Autodesk Inventor part; units mm, degrees
ref_plane "Work Plane1" through (42.6466, 0, 0) normal (1, 0, 0) x (0, 1, 0)
ref_plane "Work Plane2" through (-42.6466, 0, 0) normal (1, 0, 0) x (0, 1, 0)
ref_plane "Work Plane3" through (0, 0, -42.6466) normal (0, 0, 1) x (1, 0, 0)
sketch "Sketch1" plane through (0, 0, 0) normal (0, 0, 1) x (1, 0, 0)
  line L0 (17.5514, 0) -> (46.0756, 0)
  line L1 (46.0756, 0) -> (46.0756, 12.7)
  line L2 (46.0756, 12.7) -> (0, 12.7)
  line L3 (0, 12.7) -> (0, 0)
  line L4 (17.5514, 12.7) -> (17.5514, 0)
  line L5 (46.0756, 8.9662) -> (42.3672, 8.9662)
  line L6 (42.3672, 7.747) -> (42.3672, 0)
  line L7 (46.0756, 7.747) -> (42.3672, 7.747)
  line L8 (46.0756, 8.9662) -> (42.3672, 7.747)
  line L9 (0, 11.1252) -> (0, 12.7)
  line L10 (17.5514, 0) -> (23.85, 0)
  line L11 (0, -2.5) -> (0, 0)
  line L12 (0, 12.7) -> (38.0365, 12.7)
  line L13 (38.0365, 12.7) -> (38.0365, 14.2748)
  line L14 (38.0365, 14.2748) -> (0, 14.2748)
  line L15 (0, 14.2748) -> (0, 12.7)
  line L16 (17.5514, 12.7) -> (17.5514, 14.2748)
  line L17 (0, 0) -> (17.5514, 0)
  dimension "d1" = 12.7
  dimension "d3" = 3.7338
  dimension "d5" = 4.953
  dimension "d8" = 17.5514
  dimension "d9" = 42.3672
  dimension "d10" = 46.0756
  dimension "d11" = 1.5748
  dimension "d12" = 38.0365
revolve "Revolution1" add sketch "Sketch1" angle 360 about axis through (0, 12.7, 0) along (0, -1, 0) contours L4 L2 L1 L8 L6 L0 | L17 L3 L2 L4 | L16 L14 L13 L2 | L2 L15 L14 L16
sketch "Sketch2" plane through (0, 14.2748, 0) normal (0, 1, 0) x (1, 0, 0)
  circle A0 centre (0, 0) radius 30.1752
  point P0 (0, 30.1752)
  point P1 (0, -30.1752)
  dimension "d14" = 60.3504
hole "Hole1" at (0, 14.2748, -30.1752) at (0, 14.2748, 30.1752) direction (0, -1, 0) diameter 6.35 depth 10.16
fillet "Fillet1" radius 3.175 1 edges at (-42.3672, 0, 0)
sketch "Sketch3" plane through (0, 0, 0) normal (0, -1, 0) x (1, 0, 0)
  circle A0 centre (0, 0) radius 25.3365
  dimension "d23" = 50.673
extrude "Extrusion1" cut sketch "Sketch3" against normal blind 7.9375
sketch "Sketch5" plane through (0, 7.9375, 0) normal (0, -1, 0) x (1, 0, 0)
  line L0 (42.3672, -42.3672) -> (42.3672, 42.3672)
  line L1 (42.3672, 42.3672) -> (-42.3672, 42.3672)
  line L2 (-42.3672, 42.3672) -> (-42.3672, -42.3672)
  line L3 (-42.3672, -42.3672) -> (42.3672, -42.3672)
  line L4 (42.3672, -42.3672) -> (-42.3672, 42.3672) construction
  line L5 (42.3672, 42.3672) -> (-42.3672, -42.3672) construction
  point P0 (0, 0)
sketch "Sketch6" plane through (0, 0, 0) normal (1, 0, 0) x (0, 1, 0)
  point P0 (0, 0)
ref_plane "Work Plane1" through (42.6466, 0, 0) normal (1, 0, 0) x (0, 1, 0)
sketch "Sketch7" plane through (42.6466, 0, 0) normal (1, 0, 0) x (0, 1, 0)
  line L0 (3.175, 42.3672) -> (3.175, -42.3672)
  line L1 (3.175, 0) -> (7.7045, 0)
  point P0 (0, 0)
  point P1 (5.4398, 0)
ref_plane "Work Plane2" through (-42.6466, 0, 0) normal (1, 0, 0) x (0, 1, 0)
sketch "Sketch9" plane through (-42.6466, 0, 0) normal (1, 0, 0) x (0, 1, 0)
  line L0 (3.175, 42.3672) -> (3.175, -42.3672)
  line L1 (3.175, 0) -> (7.747, 0)
  line L2 (7.747, 42.3672) -> (7.747, -42.3672)
  point P0 (0, 0)
  point P1 (5.461, 0)
ref_plane "Work Plane3" through (0, 0, -42.6466) normal (0, 0, 1) x (1, 0, 0)
sketch "Sketch10" plane through (0, 0, -42.6466) normal (0, 0, 1) x (1, 0, 0)
  line L0 (-42.3672, 7.747) -> (42.3672, 7.747)
  line L1 (0, 7.747) -> (0, 3.175)
  line L2 (-42.3672, 3.175) -> (42.3672, 3.175)
  point P0 (0, 0)
  point P1 (0, 5.461)
ref_plane "Work Plane4" through (0, 0, 42.6466) normal (0, 0, 1) x (1, 0, 0)
sketch "Sketch11" plane through (0, 0, 42.6466) normal (0, 0, 1) x (1, 0, 0)
  line L0 (-42.3672, 3.175) -> (42.3672, 3.175)
  line L1 (0, 3.175) -> (0, 7.747)
  line L2 (-42.3672, 7.747) -> (42.3672, 7.747)
  point P0 (0, 0)
  point P1 (0, 5.461)
hole "Hole2" at (-42.6466, 5.461, 0) direction (-1, 0, 0) diameter 3.302 end through all
hole "Hole3" at (42.6466, 5.4398, 0) direction (-1, 0, 0) diameter 3.302 end through all
hole "Hole4" at (0, 5.461, 42.6466) direction (0, 0, -1) diameter 3.302 end through all
hole "Hole5" at (0, 7.9375, 0) direction (0, 1, 0) diameter 30.1625 end through all
chamfer "Chamfer1" distance 0.254 angle 45 2 edges at (-46.0756, 12.7, 0) (0, 14.2748, 15.0812)
properties part number "2016.06.09 Judson M204 Adapter" material "Aluminum 6061"
CAD build for the part. Positions are in the model's coordinates, mm. A direction names the side the tool comes from. Give positions to 0.01 mm unless a question says otherwise; leave off trailing zeros. Answer as CSV lines item,"result".
Q1. 3-axis set-ups, long thin cutter, end or side, ignore diameter. For faces 5 (the face through (-9.18, 5.43, -41.36)), 6 (the face through (-33.94, 7.05, 0.36)), 7 (the face through (2, 4.115, 30)): which of +Z, -Z, +X, -X, +Y, -Y reach the whole face in a straight line?
Result set:
face 5,"-Y"
face 6,"+X, -X"
face 7,"+Y"
Q2. Band-saw the part on A-A (z = 0). State how many separate pieces and enclosed holes the cut face has, and give its area (3 significant figures).
Result set:
separate pieces,"4"
enclosed holes,"0"
area,"518 mm²"
Q3. Flat gauge pins, fed straight in: pin 1 Ø1.1 at (x, z) = (1.5, 31) entering from +Y; pin 2 Ø3 at (y, z) = (4, -26) entering from -X; pin 3 Ø6 at (x, z) = (-12, -2.5) entering from -Y; pin 4 Ø2.5 at (x, y) = (0, 5.461) entering from -Z. Where does each tip first touch, or does it go through?
Result set:
pin 1,"y = 4.11"
pin 2,"x = -34.56"
pin 3,"y = 7.94"
pin 4,"through"
Q4. Pull direction X, two halves, no side cores. Call faces 1 (the face through (-9.99, 10.73, 44.98)), 2 (the face through (-0.663, 11.022, 15.067)), 3 (the face through (-17.2, 12.7, 34.2)), 4 (the face through (-0.496, 3.886, -35.843)): released by +X, released by -X, zero draft, split by the parting line, or undercut.
Result set:
face 1,"split by the parting line"
face 2,"undercut"
face 3,"zero draft"
face 4,"undercut"
Q5. Drill centre lines: line 1 (Z direction, x = 0, y = 9.5); line 2 (Y direction, x = 35.25, z = 0); line 3 (Y direction, x = 0, z = -39). Where is each one in solid material? Low to high. Write a range as from..to.
Result set:
line 1,"-46.08..-33.35, -27..-15.08, 15.08..27, 33.35..46.08"
line 2,"0..3.79, 7.09..14.27"
line 3,"0..3.81, 7.11..12.7"
